Part model, mm, in its own coordinate system. Face numbers are marked on the shaded views. A direction names the side the tool comes from. Give positions to 0.01 mm unless a question says otherwise; leave off trailing zeros. Write each loop counter-clockwise with the first axis right and the second up, starting at its lowest first coordinate (ties: lowest second). Pieces come first, ordered by that corner, then holes. Notation, with made-up numbers: M -28.75,-29.75 L -17.75,-29.75 A17 cw -17.75,-22.75 Z; hole C 31.25,-30 d3. An arc over 180 degrees is marked long. Use CSV: the item, a comma, the result in double quotes. Start each with the question number.
Item 1: Mould opens along X. For the marked faces 1 and 2 say: released by +X, released by -X, zero draft, split by the parting line, or undercut.
Item 2: Cut at D-D (z = 4.25). List the corners of the cut face in (x, y) (1 decimal).
Item 3: Cut at C-C (x = -22.5). List the corners of the cut face in (y, z) (3 decimals), then the cut area to 3 significant figures.
Item 4: Drill centre lines: line 1 (X direction, y = -19.75, z = 2.5); line 2 (X direction, y = -16, z = 9.75); line 3 (Y direction, x = -17.5, z = 6.25) (3 decimals). Where is each one in solid material? Low to high. Write a range as [from, to].
Item 5: Which spindle directions (+Z, -Z, +X, -X, +Y, -Y) get a long thin tool onto all of the face, cutting with end or side? Do the marked faces 3 and 4. Say none if no direction does.
Item 6: Cut at A-A (y = -17.25). List the corners of the cut face in (x, z) (1 decimal), then the cut area to 3 significant figures.
Item 7: Cut at B-B (z = 0.5). List the corners of the cut face in (x, y) (1 decimal).
Item 8: Pin check, flat tips, straight feed: pin 1 (5 mm diameter, centred on y = -18, z = 7.5, fed in from +X); pin 2 (4 mm diameter, centred on y = -16, z = 5.5, fed in from +X); pin 3 (0.6 mm diameter, centred on x = -15.5, y = -1, fed in from +Z). Stop position of each tip, or through.
from build123d import *

# Parameters (mm, degrees)
F0_R     = 1.25
F1_DEPTH = 21.875
F2_W     = 22.395833
F2_H     = 17.708334
F2_W_2   = 4.166666
F3_DEPTH = 10.417667


with BuildPart() as f1:
    # F0 (on Front) → F1 (new body)
    with BuildSketch(Plane.XZ):
        Polygon((-28.645833, 0), (0, 0), (28.645833, 0), (28.645833, 3.125), (19.8125, 3.125), (12.5, 3.125), (9.333333, 6.291667), (5.208333, 10.416667), (0, 10.416667), (-5.208333, 10.416667), (-9.333333, 6.291667), (-12.5, 3.125), (-19.8125, 3.125), (-28.645833, 3.125), align=None)
        Polygon((12.5, 3.125), (19.8125, 3.125), (19.8125, 7.770833), (18.0625, 10.020833), (13.0625, 10.020833), (9.333333, 6.291667), align=None)
        with Locations((15.5625, 7.770833)):
            Circle(F0_R, mode=Mode.SUBTRACT)
        Polygon((-19.8125, 7.770833), (-19.8125, 3.125), (-12.5, 3.125), (-9.333333, 6.291667), (-13.0625, 10.020833), (-18.0625, 10.020833), align=None)
        with Locations((-15.5625, 7.770833)):
            Circle(F0_R, mode=Mode.SUBTRACT)
    extrude(amount=F1_DEPTH)

    # F2 (on face) → F3 (cut, through all)
    with BuildSketch(Plane.XY.offset(10.416667)):
        with Locations((-15.364584, -10.9375)):
            Rectangle(F2_W, F2_H)
        with Locations((15.364584, -10.9375)):
            Rectangle(F2_W, F2_H)
        with Locations((0, -10.9375)):
            Rectangle(F2_W_2, F2_H)
    extrude(amount=-F3_DEPTH, mode=Mode.SUBTRACT)


solid = f1.part
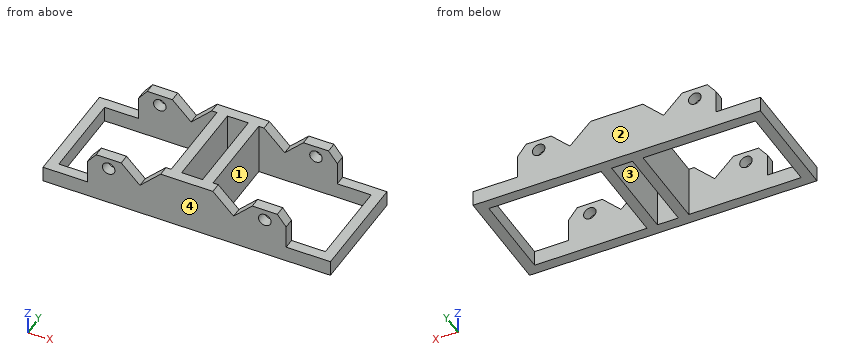
Worked answers:
1,face 1,"undercut"
1,face 2,"zero draft"
2,outline,"M -19.8,-21.9 L 19.8,-21.9 L 19.8,-19.8 L 4.2,-19.8 L 4.2,-2.1 L 19.8,-2.1 L 19.8,0 L -19.8,0 L -19.8,-2.1 L -4.2,-2.1 L -4.2,-19.8 L -19.8,-19.8 Z; hole M -2.1,-19.8 L 2.1,-19.8 L 2.1,-2.1 L -2.1,-2.1 Z"
3,outline,"M -21.875,0 L -19.792,0 L -19.792,3.125 L -21.875,3.125 Z; M -2.083,0 L 0,0 L 0,3.125 L -2.083,3.125 Z"
3,area,"13.0 mm^2"
4,line 1,"x = [-28.65, -26.56], [-4.17, -2.08], [2.08, 4.17], [26.56, 28.65]"
4,line 2,"x = [-4.17, -2.08], [2.08, 4.17]"
4,line 3,"y = [-21.875, -19.792], [-2.083, 0]"
5,face 3,"+Z, -Z"
5,face 4,"+Z, -Z, +X, -X, -Y"
6,outline,"M -28.6,0 L -26.6,0 L -26.6,3.1 L -28.6,3.1 Z; M -4.2,0 L -2.1,0 L -2.1,10.4 L -4.2,10.4 Z; M 2.1,0 L 4.2,0 L 4.2,10.4 L 2.1,10.4 Z; M 26.6,0 L 28.6,0 L 28.6,3.1 L 26.6,3.1 Z"
6,area,"56.4 mm^2"
7,outline,"M -28.6,-21.9 L 28.6,-21.9 L 28.6,0 L -28.6,0 Z; hole M -26.6,-19.8 L -4.2,-19.8 L -4.2,-2.1 L -26.6,-2.1 Z; hole M -2.1,-19.8 L 2.1,-19.8 L 2.1,-2.1 L -2.1,-2.1 Z; hole M 4.2,-19.8 L 26.6,-19.8 L 26.6,-2.1 L 4.2,-2.1 Z"
8,pin 1,"stops at x = 19.81"
8,pin 2,"stops at x = 4.17"
8,pin 3,"stops at z = 10.02"
